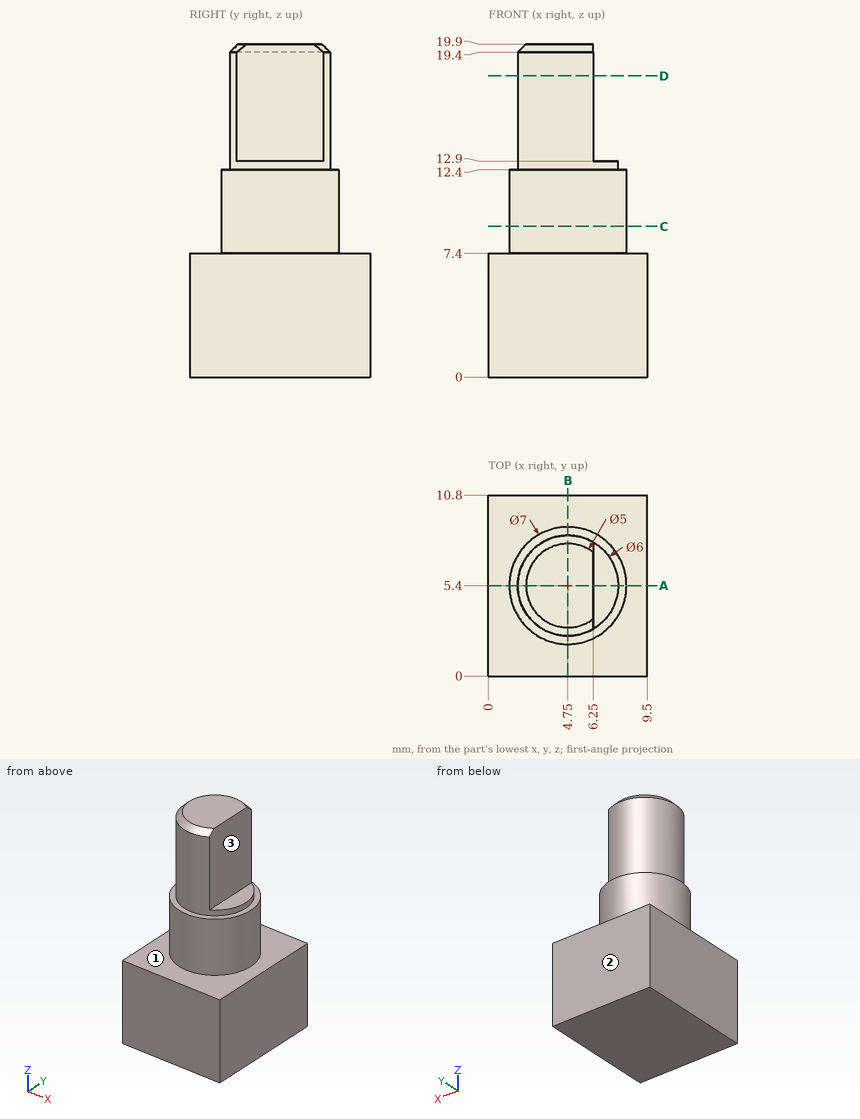
The drawing under review shows one solid part. Ordinate dimensions are in mm from its lowest x, y, z. A direction names the side the tool comes from. Coordinates: 2 decimals unless noted, no trailing zeros. Write each loop counter-clockwise with the first axis right and the second up, starting at its lowest first coordinate (ties: lowest second). Pieces come first, ordered by that corner, then holes. Notation, with made-up numbers: (44, 1) - (49, 1) arc R28 ccw to (49, 27) - close; hole circle Ø6 at (-21.5, 82). An arc over 180 degrees is marked (long way). Answer as CSV lines item,"result".
(1) We need section C-C (z = 9). Give the boundary of the cut face in (x, y), plus the area to 3 significant figures.
Data:
outline,"circle Ø7 at (4.75, 5.4)"
area,"38.5 mm2"
(2) We need section D-D (z = 18). Give the boundary of the cut face in (x, y).
Data:
outline,"(6.25, 2.8) - (6.25, 8) arc R3 ccw (long way) to start"
(3) Clearance check with flat-ended pins moving along their axes: pin 1 Ø4 at (x, z) = (4.5, 17.5) entering from -Y; pin 2 Ø1 at (x, z) = (5.5, 13) entering from +Y; pin 3 Ø2 at (y, z) = (6, 14.5) entering from +X. State where each tip first meets the part, or that it passes through.
Data:
pin 1,"stops at y = 2.4"
pin 2,"stops at y = 8.39"
pin 3,"stops at x = 6.25"
(4) Tool access review of the marked faces 1, 2 and 3: name each direction out of +Z, -Z, +X, -X, +Y, -Y from which nothing blocks a thin tool from reaching the whole face with its end or side.
Data:
face 1,"+Z"
face 2,"+Z, -Z, +X, -X, +Y"
face 3,"+Z, +X, +Y, -Y"
(5) For line 1 along Z through (x, y) = (1.75, 1); line 2 along Z through (x, y) = (6.5, 4); line 3 along X through (y, z) = (3.75, 14.5), list the stretches that pass through material, from the lowest coordinate up. Write a range as [from, to].
Data:
line 1,"z = [0, 7.4]"
line 2,"z = [0, 12.9]"
line 3,"x = [2.24, 6.25]"
(6) We need section B-B (x = 4.75). Give the boundary of the cut face in (y, z), plus the area to 3 significant figures.
Data:
outline,"(0, 0) - (10.8, 0) - (10.8, 7.4) - (8.9, 7.4) - (8.9, 12.4) - (8.4, 12.4) - (8.4, 19.4) - (7.9, 19.9) - (2.9, 19.9) - (2.4, 19.4) - (2.4, 12.4) - (1.9, 12.4) - (1.9, 7.4) - (0, 7.4) - close"
area,"160 mm2"
(7) We need section A-A (y = 5.4). Give the boundary of the cut face in (x, z).
Data:
outline,"(0, 0) - (9.5, 0) - (9.5, 7.4) - (8.25, 7.4) - (8.25, 12.4) - (7.75, 12.4) - (7.75, 12.9) - (6.25, 12.9) - (6.25, 19.9) - (2.25, 19.9) - (1.75, 19.4) - (1.75, 12.4) - (1.25, 12.4) - (1.25, 7.4) - (0, 7.4) - close"
